```python
from build123d import *

# Parameters (mm, degrees)
SKETCH1_W                = 35
SKETCH1_H                = 40
BOSS_EXTRUDE1_DEPTH      = 3
SKETCH2_R                = 12.6
CUT_EXTRUDE1_DEPTH       = 27.744158241
SKETCH4_W                = 35
SKETCH4_H                = 3
BOSS_EXTRUDE2_DEPTH      = 23.5
SKETCH5_W                = 35
SKETCH5_H                = 80
BOSS_EXTRUDE3_DEPTH      = 3
SKETCH6_W                = 35
SKETCH6_H                = 63.5
SKETCH6_R                = 12.6
BOSS_EXTRUDE4_DEPTH      = 3
BOSS_EXTRUDE5_DEPTH      = 10
BOSS_EXTRUDE5_DEPTH_BACK = 13
SKETCH7_W                = 35
SKETCH7_H                = 3
FILLET1_R                = 5
SKETCH8_W                = 100
SKETCH8_H                = 30
BOSS_EXTRUDE6_DEPTH      = 3
SKETCH10_W               = 100
SKETCH10_H               = 2
BOSS_EXTRUDE8_DEPTH      = 3
SKETCH12_R               = 1.5
CUT_EXTRUDE3_DEPTH       = 108.801901653
MIRROR2_COPY_1_SKETCH_R  = 1.5
MIRROR2_COPY_1_DEPTH     = 108.801901653
CUT_EXTRUDE4_DEPTH       = 32.5
SKETCH26_R               = 1.5
CUT_EXTRUDE17_DEPTH      = 10


with BuildPart() as part:
    # Sketch1 → Boss-Extrude1 (new body)
    with BuildSketch(Plane(origin=(0, 0, 0), x_dir=(1, 0, 0), z_dir=(0, 1, 0))):
        Rectangle(SKETCH1_W, SKETCH1_H)
    extrude(amount=BOSS_EXTRUDE1_DEPTH)

    # Sketch2 → Cut-Extrude1 (cut, through all)
    with BuildSketch(Plane(origin=(0, 3, 0), x_dir=(1, 0, 0), z_dir=(0, 1, 0))):
        with Locations(Location((0, 0, 0), (0, 0, 270))):
            Circle(SKETCH2_R)
    extrude(amount=-CUT_EXTRUDE1_DEPTH, mode=Mode.SUBTRACT)

    # Sketch4 → Boss-Extrude2 (add)
    with BuildSketch(Plane(origin=(0, 0, -20), x_dir=(-1, 0, 0), z_dir=(0, 0, -1))):
        with Locations((0, 1.5)):
            Rectangle(SKETCH4_W, SKETCH4_H)
    extrude(amount=BOSS_EXTRUDE2_DEPTH)

    # Sketch5 → Boss-Extrude3 (add)
    with BuildSketch(Plane(origin=(0, 0, -43.5), x_dir=(-1, 0, 0), z_dir=(0, 0, -1))):
        with Locations((0, -37)):
            Rectangle(SKETCH5_W, SKETCH5_H)
    extrude(amount=BOSS_EXTRUDE3_DEPTH)

    # Sketch6 → Boss-Extrude4 (add)
    with BuildSketch(Plane(origin=(0, -17, 0), x_dir=(1, 0, 0), z_dir=(0, 1, 0))):
        with Locations((0, 11.75)):
            Rectangle(SKETCH6_W, SKETCH6_H)
        with Locations(Location((0, 0, 0), (0, 0, 270))):
            Circle(SKETCH6_R, mode=Mode.SUBTRACT)
    extrude(amount=-BOSS_EXTRUDE4_DEPTH)

    # Sketch7 → Boss-Extrude5 (add, two sides: drawn at the far end of the back side and taken through both)
    with BuildSketch(Plane.XY.offset(-43.5).offset(-BOSS_EXTRUDE5_DEPTH_BACK)):
        with Locations((0, -75.5)):
            Rectangle(SKETCH7_W, SKETCH7_H)
    extrude(amount=BOSS_EXTRUDE5_DEPTH + BOSS_EXTRUDE5_DEPTH_BACK)

    # Fillet1
    fillet1_edges = [part.edges().sort_by_distance(p)[0] for p in [
        (0, 0, -43.5),
        (0, -20, -43.5),
        (0, -17, -43.5),
        (0, -74, -46.5),
        (0, -74, -43.5),
    ]]
    fillet(fillet1_edges, radius=FILLET1_R)

    # Sketch8 → Boss-Extrude6 (add)
    with BuildSketch(Plane.XY.offset(-43.5)):
        with Locations((0, -51)):
            Rectangle(SKETCH8_W, SKETCH8_H)
    extrude(amount=-BOSS_EXTRUDE6_DEPTH)

    # Sketch10 → Boss-Extrude8 (add)
    with BuildSketch(Plane.XY.offset(-43.5)):
        with Locations((0, -47)):
            Rectangle(SKETCH10_W, SKETCH10_H)
        with Locations((0, -55)):
            Rectangle(SKETCH10_W, SKETCH10_H)
    extrude(amount=BOSS_EXTRUDE8_DEPTH)

    # Sketch12 → Cut-Extrude3 (cut, through all)
    with BuildSketch(Plane(origin=(0, -74, 0), x_dir=(1, 0, 0), z_dir=(0, 1, 0))):
        with Locations(Location((-13.5, 36.5, 0), (0, 0, 270))):
            Circle(SKETCH12_R)
    cut_extrude3 = extrude(amount=-CUT_EXTRUDE3_DEPTH, mode=Mode.SUBTRACT)

    # Mirror1: Cut-Extrude3 across plane
    add(cut_extrude3.mirror(Plane.ZY), mode=Mode.SUBTRACT)

    # Mirror2: Cut-Extrude3 across plane
    add(cut_extrude3.mirror(Plane(origin=(0, 0, -45), x_dir=(1, 0, 0), z_dir=(0, 0, -1))), mode=Mode.SUBTRACT)

    # Mirror2 copy 1 sketch → Mirror2 copy 1 (cut, through all)
    with BuildSketch(Plane(origin=(0, -74, -90), x_dir=(-1, 0, 0), z_dir=(0, 1, 0))):
        with Locations(Location((-13.5, 36.5, 0), (0, 0, 270))):
            Circle(MIRROR2_COPY_1_SKETCH_R)
    extrude(amount=-MIRROR2_COPY_1_DEPTH, mode=Mode.SUBTRACT)

    # Sketch13 → Cut-Extrude4 (cut)
    with BuildSketch(Plane.ZY.offset(50)):
        Polygon((-43.5, -36), (-46.5, -36), (-46.5, -66), (-43.5, -66), (-43.5, -56), (-40.5, -56), (-40.5, -54), (-43.5, -54), (-43.5, -48), (-40.5, -48), (-40.5, -46), (-43.5, -46), align=None)
    extrude(amount=-CUT_EXTRUDE4_DEPTH, mode=Mode.SUBTRACT)

    # Sketch26 → Cut-Extrude17 (cut)
    with BuildSketch(Plane(origin=(0, 3, 0), x_dir=(1, 0, 0), z_dir=(0, 1, 0))):
        with Locations(Location((0, 26.5, 0), (0, 0, 270))):
            Circle(SKETCH26_R)
    extrude(amount=-CUT_EXTRUDE17_DEPTH, mode=Mode.SUBTRACT)


solid = part.part
```
The model under review builds one solid part; all positions refer to its coordinate system, in mm. A direction names the side the tool comes from. Round coordinates to 2 decimals unless told otherwise and drop trailing zeros. Order: outer loops, then holes, each group sorted by start corner. A loop starts at its lowest first (then second) coordinate and runs counter-clockwise, first axis right, second up.
Item 1: Add section A-A, the plane z = -26.5. State the section outline as (x, y) points, and give its area (3 significant figures).
Working result:
outline: (-17.5, -20) - (17.5, -20) - (17.5, -17) - (-17.5, -17) - close; (-17.5, 0) - (-1.5, 0) - (-1.5, 3) - (-17.5, 3) - close; (1.5, 0) - (17.5, 0) - (17.5, 3) - (1.5, 3) - close
area: 201 mm2
Item 2: To check wall thickness, follow probe 1 along X at (y, z) = (-76, -53); probe 2 along Y at (x, z) = (14, -32); probe 3 along Y at (x, z) = (-6, -40). State the ranges of each line that lie inside material, in increasing order.
Working result:
probe 1: x = -17.5 to -14.91, -12.09 to 12.09, 14.91 to 17.5
probe 2: y = -20 to -17, 0 to 3
probe 3: y = -77 to -73.77, -20.23 to -16.77, -0.23 to 3
Item 3: Machinability: for faces 1 (the cylindrical face through (14.4, -75.5, -37.7)), 2 (the flat face through (0, -8, -43.5)), 3 (the flat face through (34, -66, -45)), 4 (the flat face through (17.5, -18, -21)), which of the approach directions +Z, -Z, +X, -X, +Y, -Y give a long, thin tool a straight path to every point of the face, cutting with its end or side? Answer none if there is none.
Working result:
face 1: -Y
face 2: +Z, +X, -X
face 3: +Z, -Z, +X, -Y
face 4: +Z, -Z, +X, +Y
Item 4: Add section B-B, the plane z = 0. State the section outline as (x, y) points.
Working result:
outline: (-17.5, -20) - (-12.6, -20) - (-12.6, -17) - (-17.5, -17) - close; (-17.5, 0) - (-12.6, 0) - (-12.6, 3) - (-17.5, 3) - close; (12.6, -20) - (17.5, -20) - (17.5, -17) - (12.6, -17) - close; (12.6, 0) - (17.5, 0) - (17.5, 3) - (12.6, 3) - close
Item 5: Add section C-C, the plane x = 28. State the section outline as (y, z) points, and give its area (3 significant figures).
Working result:
outline: (-66, -46.5) - (-36, -46.5) - (-36, -43.5) - (-46, -43.5) - (-46, -40.5) - (-48, -40.5) - (-48, -43.5) - (-54, -43.5) - (-54, -40.5) - (-56, -40.5) - (-56, -43.5) - (-66, -43.5) - close
area: 102 mm2
Item 6: Draft analysis for pull direction Z (two halves, no side actions). For faces 5 (the cylindrical face through (-14.4, -75.5, -37.7)), 6 (the cylindrical face through (0.25, -72.5, -42.07)), 7 (the flat face through (8, -40, -46.5)), 8 (the flat face through (16, -48, -42)), state which applies: released by +Z, released by -Z, zero draft, split by the parting line, or undercut.
Working result:
face 5: undercut
face 6: released by +Z
face 7: released by -Z
face 8: zero draft
Item 7: Add section D-D, the plane z = -15. State the section outline as (x, y) points.
Working result:
outline: (-17.5, -20) - (17.5, -20) - (17.5, -17) - (-17.5, -17) - close; (-17.5, 0) - (17.5, 0) - (17.5, 3) - (-17.5, 3) - close
Item 8: For pin 1 (1.5 mm diameter, centred on x = 26.5, z = -45.5, fed in from -Y); pin 2 (15 mm diameter, centred on x = 0, z = 0, fed in from -Y); pin 3 (6 mm diameter, centred on x = 24, y = -68.5, fed in from -Z); pin 4 (17 mm diameter, centred on x = 3.5, y = -40.5, fed in from +Z), all flat-tipped, find the tip position at first contact; note any pin that passes through.
Working result:
pin 1: stops at y = -66
pin 2: passes through
pin 3: stops at z = -46.5
pin 4: stops at z = -40.5
